```python
from build123d import *

# Parameters (mm, degrees)
SKETCH3_R                = 10
SKETCH3_R_2              = 6.5
BOSS_EXTRUDE1_DEPTH      = 1.1
BOSS_EXTRUDE1_DEPTH_BACK = 1.1
FILLET1_R                = 0.4
FILLET2_R                = 0.1


with BuildPart() as part:
    # Sketch3 → Boss-Extrude1 (new body, two sides)
    with BuildSketch(Plane.XY) as boss_extrude1_sk:
        Circle(SKETCH3_R)
        Circle(SKETCH3_R_2, mode=Mode.SUBTRACT)
    extrude(amount=BOSS_EXTRUDE1_DEPTH)
    extrude(boss_extrude1_sk.sketch, amount=-BOSS_EXTRUDE1_DEPTH_BACK)

    # Fillet1
    fillet1_edges = [part.edges().sort_by_distance(p)[0] for p in [
        (-10, 0, 1.1),
        (-6.5, 0, 1.1),
    ]]
    fillet(fillet1_edges, radius=FILLET1_R)

    # Fillet2
    fillet2_edges = [part.edges().sort_by_distance(p)[0] for p in [
        (-10, 0, -1.1),
        (-6.5, 0, -1.1),
    ]]
    fillet(fillet2_edges, radius=FILLET2_R)


solid = part.part
```
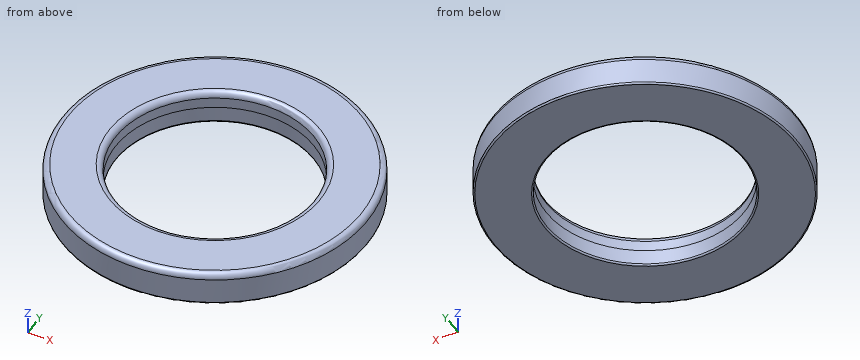
Input: part model. Units: mm. Frame: model coordinates. Round coordinates to 2 decimals unless told otherwise and drop trailing zeros. Loops run counter-clockwise (first coordinate to the right, second up) from the corner with the lowest first, then second, coordinate; pieces in that order, holes last. Notation, with made-up numbers: M -29.5,79 L 2.5,79 A25 cw 2.5,108 Z; hole C 45.25,42 d2. An arc over 180 degrees is marked long. Answer in a Markdown table with one row per item. Add a question column.
1. Ray query, probe 1 along Y at (x, z) = (0, 0.25); probe 2 along X at (y, z) = (-5.75, 0.25); probe 3 along Y at (x, z) = (1.75, -0.15). Return the intervals inside material, ascending.
2. Section C-C (z = 0.3). Output: boundary loops of the cut face in (x, y), and give its area (3 significant figures).
3. Section A-A (x = 0). Output: boundary loops of the cut face in (y, z), and give its area (3 significant figures).
4. Contact query for a flat-ended pin moving along its axis: pin 1 (10.5 mm diameter, centred on x = 0, y = 0, fed in from -Z). Output: stop coordinate, or through.
Values follow:
| question | item | result |
|---|---|---|
| 1 | probe 1 | -10 to -6.5, 6.5 to 10 |
| 1 | probe 2 | -8.18 to -3.03, 3.03 to 8.18 |
| 1 | probe 3 | -9.85 to -6.26, 6.26 to 9.85 |
| 2 | outline | C 0,0 d20; hole C 0,0 d13 |
| 2 | area | 181 mm^2 |
| 3 | outline | M -10,-1 A0.1 ccw -9.9,-1.1 L -6.6,-1.1 A0.1 ccw -6.5,-1 L -6.5,0.7 A0.4 ccw -6.9,1.1 L -9.6,1.1 A0.4 ccw -10,0.7 Z; M 6.5,-1 A0.1 ccw 6.6,-1.1 L 9.9,-1.1 A0.1 ccw 10,-1 L 10,0.7 A0.4 ccw 9.6,1.1 L 6.9,1.1 A0.4 ccw 6.5,0.7 Z |
| 3 | area | 15.3 mm^2 |
| 4 | pin 1 | through |
